The listing builds one solid part. Answer for the finished solid, in the listing's coordinates (mm). Round coordinates to 2 decimals unless told otherwise and drop trailing zeros. Write each loop counter-clockwise with the first axis right and the second up, starting at its lowest first coordinate (ties: lowest second). Pieces come first, ordered by that corner, then holes. Notation, with made-up numbers: (47, -33) - (52, -33) arc R18 ccw to (52, -15) - close; hole circle Ø1 at (78, 85.5). An arc over 180 degrees is marked (long way). Answer in a Markdown table with one row per item.
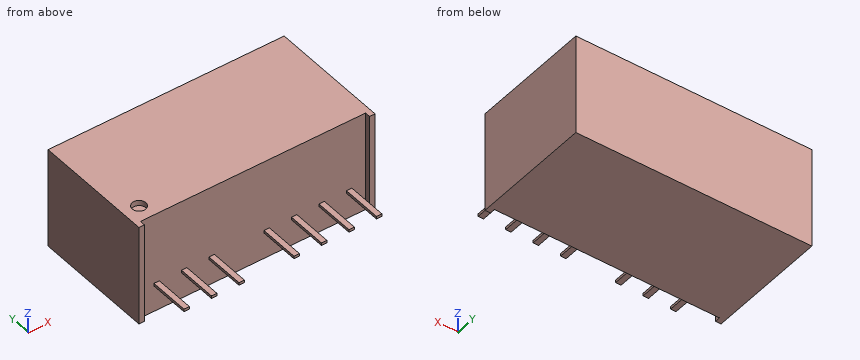
from build123d import *

# Parameters (mm, degrees)
BOSS_EXTRUDE1_DEPTH = 9.3
SKETCH3_W           = 0.5
SKETCH3_H           = 0.25
BOSS_EXTRUDE2_DEPTH = 3.7
SKETCH4_R           = 0.625
CUT_EXTRUDE1_DEPTH  = 0.5


with BuildPart() as part:
    # Sketch2 → Boss-Extrude1 (new body)
    with BuildSketch(Plane.XY):
        Polygon((0, 0), (0, 11.2), (21.8, 11.2), (21.8, 0), (21.3, 0), (21.3, 0.5), (0.5, 0.5), (0.5, 0), align=None)
    extrude(amount=BOSS_EXTRUDE1_DEPTH)

    # Sketch3 → Boss-Extrude2 (add)
    with BuildSketch(Plane.XZ.offset(-0.5)):
        with Locations((2, 2.575)):
            Rectangle(SKETCH3_W, SKETCH3_H)
        with Locations((4.54, 2.575)):
            Rectangle(SKETCH3_W, SKETCH3_H)
        with Locations((7.08, 2.575)):
            Rectangle(SKETCH3_W, SKETCH3_H)
        with Locations((12.16, 2.575)):
            Rectangle(SKETCH3_W, SKETCH3_H)
        with Locations((14.7, 2.575)):
            Rectangle(SKETCH3_W, SKETCH3_H)
        with Locations((17.24, 2.575)):
            Rectangle(SKETCH3_W, SKETCH3_H)
        with Locations((19.78, 2.575)):
            Rectangle(SKETCH3_W, SKETCH3_H)
    extrude(amount=BOSS_EXTRUDE2_DEPTH)

    # Sketch4 → Cut-Extrude1 (cut)
    with BuildSketch(Plane.XY.offset(9.3)):
        with Locations((1.5, 2)):
            Circle(SKETCH4_R)
    extrude(amount=-CUT_EXTRUDE1_DEPTH, mode=Mode.SUBTRACT)


solid = part.part
(1) Section A-A (z = 2) is taken. Give the vertices of the cut face in (x, y), and give its area (3 significant figures).
Checked values:
| item | result |
|---|---|
| outline | (0, 0) - (0.5, 0) - (0.5, 0.5) - (21.3, 0.5) - (21.3, 0) - (21.8, 0) - (21.8, 11.2) - (0, 11.2) - close |
| area | 234 mm2 |
(2) Section C-C (x = 11.5) is taken. Give the vertices of the cut face in (y, z), and give its area (3 significant figures).
Checked values:
| item | result |
|---|---|
| outline | (0.5, 0) - (11.2, 0) - (11.2, 9.3) - (0.5, 9.3) - close |
| area | 99.5 mm2 |
(3) Section B-B (x = 1.5) is taken. Give the vertices of the cut face in (y, z) (3 decimals).
Checked values:
| item | result |
|---|---|
| outline | (0.5, 0) - (11.2, 0) - (11.2, 9.3) - (2.625, 9.3) - (2.625, 8.8) - (1.375, 8.8) - (1.375, 9.3) - (0.5, 9.3) - close |
(4) Find the intervals of material crossed by line 1 (Y direction, x = 1.5, z = 9.25) (3 decimals); line 2 (X direction, y = 0.25, z = 3.5); line 3 (Y direction, x = 17.25, z = 8.5), in increasing order.
Checked values:
| item | result |
|---|---|
| line 1 | y = 0.5 to 1.375, 2.625 to 11.2 |
| line 2 | x = 0 to 0.5, 21.3 to 21.8 |
| line 3 | y = 0.5 to 11.2 |
(5) Flat-ended cylindrical pins translate along their axes: pin 1 (1.1 mm diameter, centred on x = 1.5, y = 2, fed in from +Z); pin 2 (3 mm diameter, centred on y = 0, z = 5.5, fed in from -X); pin 3 (4 mm diameter, centred on x = 19, z = 6, fed in from -Y). Find the tip coordinate at first contact, or state that the pin passes through.
Checked values:
| item | result |
|---|---|
| pin 1 | stops at z = 8.8 |
| pin 2 | stops at x = 0 |
| pin 3 | stops at y = 0.5 |
